Part model, mm, in its own coordinate system. Round coordinates to 2 decimals unless told otherwise and drop trailing zeros. Loops run counter-clockwise (first coordinate to the right, second up) from the corner with the lowest first, then second, coordinate; pieces in that order, holes last.
(1) Cut at D-D on x = 46.5. List the corners of the cut face in (y, z), then the cut area to 3 significant figures.
(2) Flat gauge pin, fed straight in: pin 1 (8.5 mm diameter, centred on x = -23.55, z = -23.55, fed in from +Y). Where does the tip first touch, or does it go through?
(3) Cut at A-A on z = 30. List the corners of the cut face in (x, y), then the cut area to 3 significant figures.
(4) Mould opens along Z. For faces 1 (the face through (-65, 1, 1)), 2 (the face through (-1, 1, 45)), 3 (the face through (-1, 1, -45)), 4 (the face through (-25.857, 1.521, -22.35)) say: +Z half, -Z half, draft (parallel to the pull), parting line (faces both ways), or undercut.
(5) Cut at C-C on y = 2.25. Count the separate pieces of the cut face and the enclosed holes in it, then the cut area to 3 significant figures.
(6) Probe probe 1 along X at (y, z) = (2, 23.55); probe 2 along X at (y, z) = (1.75, 30); probe 3 along X at (y, z) = (2.75, -4.5). List the from-to ranges inside material, lowest first.
(7) Cut at B-B on x = -23.55. List the corners of the cut face in (y, z).
from build123d import *

# Parameters (mm, degrees)
SKETCH1_W           = 130
SKETCH1_H           = 90
BOSS_EXTRUDE1_DEPTH = 3
SKETCH2_R           = 2.6
CUT_EXTRUDE1_DEPTH  = 10
SKETCH3_R           = 1.5
CUT_EXTRUDE2_DEPTH  = 10
SKETCH4_R           = 6
CUT_EXTRUDE3_DEPTH  = 10


with BuildPart() as part:
    # Sketch1 → Boss-Extrude1 (new body)
    with BuildSketch(Plane(origin=(0, 0, 0), x_dir=(1, 0, 0), z_dir=(0, 1, 0))):
        Rectangle(SKETCH1_W, SKETCH1_H)
    extrude(amount=BOSS_EXTRUDE1_DEPTH)

    # Sketch2 → Cut-Extrude1 (cut)
    with BuildSketch(Plane(origin=(0, 3, 0), x_dir=(1, 0, 0), z_dir=(0, 1, 0))):
        with Locations(Location((23.55, -23.55, 0), (0, 0, 270))):
            Circle(SKETCH2_R)
        with Locations(Location((-23.55, -23.55, 0), (0, 0, 270))):
            Circle(SKETCH2_R)
        with Locations(Location((-23.55, 23.55, 0), (0, 0, 270))):
            Circle(SKETCH2_R)
        with Locations(Location((23.55, 23.55, 0), (0, 0, 270))):
            Circle(SKETCH2_R)
    extrude(amount=-CUT_EXTRUDE1_DEPTH, mode=Mode.SUBTRACT)

    # Sketch3 → Cut-Extrude2 (cut)
    with BuildSketch(Plane.XZ):
        with Locations(Location((46.5, 30, 0), (0, 0, 270))):
            Circle(SKETCH3_R)
        with Locations(Location((-46.5, 30, 0), (0, 0, 270))):
            Circle(SKETCH3_R)
        with Locations(Location((-57.5, -5.5, 0), (0, 0, 270))):
            Circle(SKETCH3_R)
        with Locations(Location((57.5, -5.5, 0), (0, 0, 270))):
            Circle(SKETCH3_R)
    extrude(amount=-CUT_EXTRUDE2_DEPTH, mode=Mode.SUBTRACT)

    # Sketch4 → Cut-Extrude3 (cut)
    with BuildSketch(Plane.XZ):
        with Locations(Location((0, 0, 0), (0, 0, 270))):
            Circle(SKETCH4_R)
    extrude(amount=-CUT_EXTRUDE3_DEPTH, mode=Mode.SUBTRACT)


solid = part.part
Final values:
1. outline: (0, -45) - (3, -45) - (3, 28.5) - (0, 28.5) - close; (0, 31.5) - (3, 31.5) - (3, 45) - (0, 45) - close
1. area: 261 mm2
2. pin 1: stops at y = 3
3. outline: (-65, 0) - (-48, 0) - (-48, 3) - (-65, 3) - close; (-45, 0) - (45, 0) - (45, 3) - (-45, 3) - close; (48, 0) - (65, 0) - (65, 3) - (48, 3) - close
3. area: 372 mm2
4. face 1: draft
4. face 2: +Z half
4. face 3: -Z half
4. face 4: undercut
5. separate pieces: 1
5. enclosed holes: 9
5. area: 11,500 mm2
6. probe 1: x = -65 to -26.15, -20.95 to 20.95, 26.15 to 65
6. probe 2: x = -65 to -48, -45 to 45, 48 to 65
6. probe 3: x = -65 to -58.62, -56.38 to -3.97, 3.97 to 56.38, 58.62 to 65
7. outline: (0, -45) - (3, -45) - (3, -26.15) - (0, -26.15) - close; (0, -20.95) - (3, -20.95) - (3, 20.95) - (0, 20.95) - close; (0, 26.15) - (3, 26.15) - (3, 45) - (0, 45) - close
